The listing builds one solid part. Answer for the finished solid, in the listing's coordinates (mm). Face numbers are marked on the shaded views. A direction names the side the tool comes from. Round coordinates to 2 decimals unless told otherwise and drop trailing zeros. Write each loop counter-clockwise with the first axis right and the second up, starting at its lowest first coordinate (ties: lowest second). Pieces come first, ordered by that corner, then holes. Notation, with made-up numbers: (63, 14.25) - (116, 14.25) arc R7 ccw to (116, 19.25) - close; hole circle Ø9 at (22.5, 79.25). An arc over 180 degrees is marked (long way). Return JSON: item names as keys, results as strings. Group by question number.
(1) Section C-C, the plane y = 17.5 is taken. Write down the section's boundary in (x, z).
(2) Each of these flat-tipped pins is pushed along its axis until it touches: pin 1 (5 mm diameter, centred on x = -56.5, z = 30.5, fed in from -Y); pin 2 (6 mm diameter, centred on y = 32, z = -41.5, fed in from +X); pin 3 (17.5 mm diameter, centred on x = 11.5, z = -2.5, fed in from +Y); pin 4 (10 mm diameter, centred on x = -4, y = 15.5, fed in from -Z). Where does it stop, or does it pass through?
(3) Which of the six approach directions +Z, -Z, +X, -X, +Y, -Y give full straight-line access (tool end or side, diameter ignored) to the marked faces 1, 2, 3, 4 and 5?
(4) Section A-A, the plane z = 0 is taken. Write down the section's boundary in (x, y), then the cut area to 3 significant figures.
(5) Section B-B, the plane y = 58.5 is taken. Write down the section's boundary in (x, z), then the cut area to 3 significant figures.
(6) Find the intervals of material crossed by line 1 along Y through (x, z) = (-17, -5.5); line 2 along X through (y, z) = (4.5, 1.5); line 3 along Y through (x, z) = (-12, -29.5), in increasing order. Write a range as [from, to].
```python
from build123d import *

# Parameters (mm, degrees)
EXTRUDE_1_REACH = 133.166


with BuildPart() as part:
    # Эскиз1 → Повернуть1 (revolve)
    with BuildSketch(Plane.XY, mode=Mode.PRIVATE) as revolve_1_sk:
        Polygon((0, 0), (-73.5, 0), (-73.5, 29), (-29, 55), (0, 55), align=None)
    revolve(revolve_1_sk.sketch.rotate(Axis((0, 0, 0), (0, -1, 0)), 270), axis=Axis((0, 0, 0), (0, -1, 0)))

    # Бобышка-Вытянуть1: up to this cone (the profile starts outside it)
    extrude_1_end = Plane(origin=(0, 80, 0), z_dir=(0, -1, 0)).offset(8.056180775) * Cone(1.712e-06, 214.986038462, 125.609819225, align=(Align.CENTER, Align.CENTER, Align.MIN), mode=Mode.PRIVATE)
    # Эскиз2 → Бобышка-Вытянуть1 (add, up to the surface)
    with BuildSketch(Plane(origin=(0, 80, 0), x_dir=(-1, 0, 0), z_dir=(0, -1, 0)), mode=Mode.PRIVATE) as extrude_1_sk1:
        with BuildLine():
            ThreePointArc((39.826891471, -50.018998092), (61.845069439, 2.908427791), (45.380271287, 57.817652822))
            ThreePointArc((45.380271287, 57.817652822), (34.438558368, 64.93254729), (22.410934831, 70))
            ThreePointArc((22.410934831, 70), (34.25441727, 33.17194105), (28.549688681, -5.090704886))
            ThreePointArc((28.549688681, -5.090704886), (20.626062909, -17.288589905), (10, -27.221315178))
            ThreePointArc((10, -27.221315178), (16.632121962, -39.182164271), (25, -50))
            ThreePointArc((25, -50), (32.409231762, -53.29825711), (39.826891471, -50.018998092))
        make_face()
    extrude_1_tool1 = extrude(extrude_1_sk1.sketch, amount=EXTRUDE_1_REACH, mode=Mode.PRIVATE) - extrude_1_end
    add(extrude_1_tool1.solids().sort_by_distance((-40.446865, 80, -0.64775))[0])


solid = part.part
```
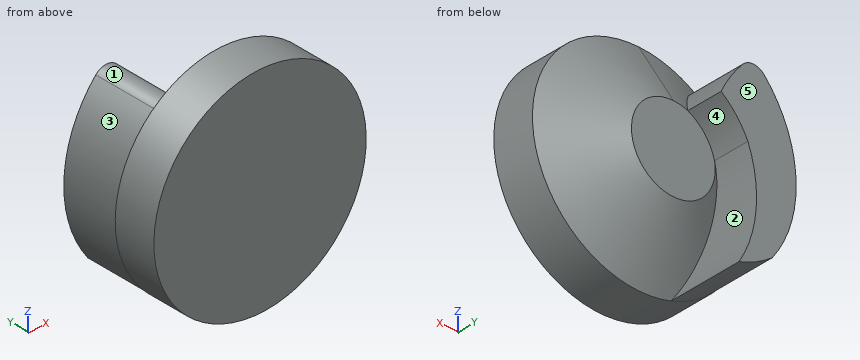
Working result:
{
 "1": {"outline": "circle Ø147 at (0, 0)"},
 "2": {"pin 1": "stops at y = 0", "pin 2": "stops at x = 60.99", "pin 3": "stops at y = 55", "pin 4": "stops at z = -73.5"},
 "3": {"face 1": "+Z, +Y", "face 2": "+Y", "face 3": "-X, +Y", "face 4": "+X, +Y", "face 5": "+Z, -Z, +X, -X, +Y"},
 "4": {"outline": "(-73.5, 0) - (73.5, 0) - (73.5, 29) - (29, 55) - (-29, 55) - (-30.38, 54.19) - (-30.38, 80) - (-61.65, 80) - (-61.65, 35.93) - (-73.5, 29) - close", "area": "8,020 mm^2"},
 "5": {"outline": "(-45.38, -57.82) arc R73.5 ccw to (-22.41, -70) arc R85 cw to (-28.55, 5.09) arc R60 cw to (-10, 27.22) arc R90 ccw to (-25, 50) arc R10 ccw to (-39.83, 50.02) arc R85.28 ccw to start", "area": "3,280 mm^2"},
 "6": {"line 1": "y = [0, 55]", "line 2": "x = [-73.48, 73.48]", "line 3": "y = [0, 53.34]"}
}
